from build123d import *

# Parameters (mm, degrees)
F0_W     = 900
F0_H     = 800
F1_DEPTH = 400
F2_W     = 400
F2_H     = 800
F3_DEPTH = 1000


with BuildPart() as f1:
    # F0 (on Top) → F1 (new body)
    with BuildSketch(Plane.XY):
        with Locations((-22.583289, 100.151006)):
            Rectangle(F0_W, F0_H)
    extrude(amount=-F1_DEPTH)

    # F2 (on face) → F3 (join)
    with BuildSketch(Plane(origin=(0, 0, -400), x_dir=(1, 0, 0), z_dir=(0, 0, -1))):
        with Locations((627.416711, -100.151006)):
            Rectangle(F2_W, F2_H)
    extrude(amount=-F3_DEPTH)


solid = f1.part
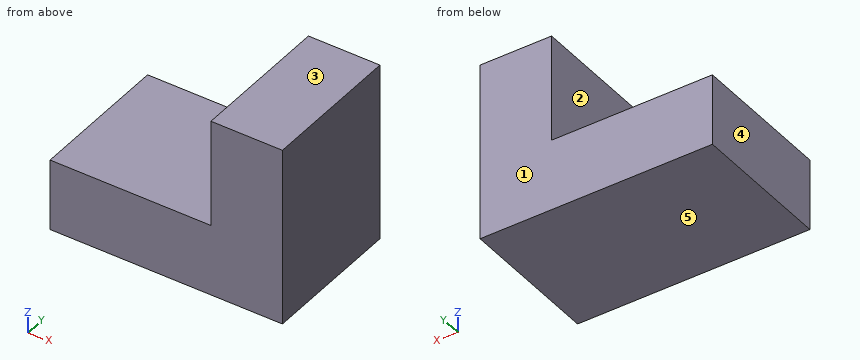
Here's how the part is built. I have some questions about the finished solid (model axes, mm). Face numbers are marked on the shaded views. A direction names the side the tool comes from. Coordinates: 2 decimals unless noted, no trailing zeros. Write each loop counter-clockwise with the first axis right and the second up, starting at its lowest first coordinate (ties: lowest second). Pieces come first, ordered by that corner, then holes.
Item 1: If I drill on line 1 (X direction, y = -141, z = 533); line 2 (Z direction, x = 421, y = -236), over which ranges is the centre line in solid material (lowest first)?
Item 2: I want a section at B-B on z = 50. Write out the boundary of the cut face in (x, y), and give its area (3 significant figures).
Item 3: Will this pin go through, and if not, where does the flat tip stop? pin 1 (12 mm diameter, centred on y = -177.5, z = 184, fed in from -X).
Item 4: On a 3-axis mill with a long thin cutter (end or side, diameter ignored), from which of +Z, -Z, +X, -X, +Y, -Y can I reach the whole of each face in a straight line? I mean the marked faces 1 and 2. Say none if no direction works.
Item 5: I want a section at A-A on y = 387. Write out the boundary of the cut face in (x, z), and give its area (3 significant figures).
Item 6: If we mould it in two halves opening along Z, with no side actions, what happens to the marked faces 3, 4 and 5? For each: +Z half, -Z half, draft (parallel to the pull), parting line (faces both ways), or undercut.
Item 7: I want a section at C-C on x = 133. Write out the boundary of the cut face in (y, z), and give its area (3 significant figures).
Findings below:
1. line 1: x = 427.42 to 827.42
1. line 2: z = -400 to 0
2. outline: (427.42, -299.85) - (827.42, -299.85) - (827.42, 500.15) - (427.42, 500.15) - close
2. area: 320,000 mm2
3. pin 1: stops at x = 427.42
4. face 1: +Z, -Z, +X, -X, +Y
4. face 2: +Z, -X, +Y, -Y
5. outline: (-472.58, -400) - (827.42, -400) - (827.42, 600) - (427.42, 600) - (427.42, 0) - (-472.58, 0) - close
5. area: 760,000 mm2
6. face 3: +Z half
6. face 4: draft
6. face 5: -Z half
7. outline: (-299.85, -400) - (500.15, -400) - (500.15, 0) - (-299.85, 0) - close
7. area: 320,000 mm2
